Work out the finished part from the listing and answer in its coordinate system (mm). Face numbers are marked on the shaded views. A direction names the side the tool comes from. Round coordinates to 2 decimals unless told otherwise and drop trailing zeros. Loops run counter-clockwise (first coordinate to the right, second up) from the corner with the lowest first, then second, coordinate; pieces in that order, holes last. Notation, with made-up numbers: (-7.5, -6.75) - (21.5, -6.75) arc R26 cw to (21.5, 28.25) - close; hole circle Ø6 at (77, 3). An arc over 180 degrees is marked (long way). Answer as CSV lines item,"result". Start each with the question number.
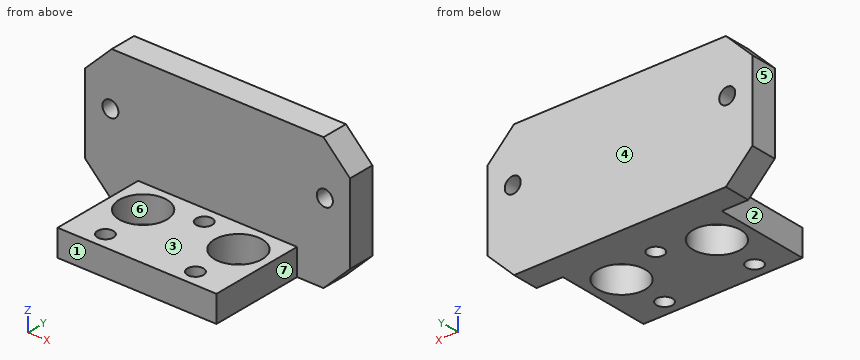
```python
from build123d import *

# Parameters (mm, degrees)
F0_R      = 1.51
F0_R_2    = 4.5
F1_DEPTH  = 5
F2_W      = 30
F2_H      = 5
F3_DEPTH  = 20
F4_W      = 5
F4_H      = 25
F5_DEPTH  = 10
F6_W      = 5
F6_H      = 25
F7_DEPTH  = 10
F9_DEPTH  = 5.001
F10_R     = 1.51
F11_DEPTH = 5.001


with BuildPart() as f1:
    # F0 (on Top) → F1 (new body)
    with BuildSketch(Plane.XY):
        Polygon((0, 18), (0, 0), (30, 0), (30, 18), (30, 23), (29.759806, 23), (0, 23), align=None)
        with Locations((6.5, 3)):
            Circle(F0_R, mode=Mode.SUBTRACT)
        with Locations((23.5, 3)):
            Circle(F0_R, mode=Mode.SUBTRACT)
        with Locations((6, 12)):
            Circle(F0_R_2, mode=Mode.SUBTRACT)
        with Locations((15, 15)):
            Circle(F0_R, mode=Mode.SUBTRACT)
        with Locations((24, 12)):
            Circle(F0_R_2, mode=Mode.SUBTRACT)
    extrude(amount=F1_DEPTH)

    # F2 (on face) → F3 (join)
    with BuildSketch(Plane.XY.offset(5)):
        with Locations((15, 20.5)):
            Rectangle(F2_W, F2_H)
    extrude(amount=F3_DEPTH)

    # F4 (on face) → F5 (join)
    with BuildSketch(Plane(origin=(0, 0, 0), x_dir=(0, -1, 0), z_dir=(-1, 0, 0))):
        with Locations((-20.5, 12.5)):
            Rectangle(F4_W, F4_H)
    extrude(amount=F5_DEPTH)

    # F6 (on face) → F7 (join)
    with BuildSketch(Plane.YZ.offset(30)):
        with Locations((20.5, 12.5)):
            Rectangle(F6_W, F6_H)
    extrude(amount=F7_DEPTH)

    # F8 (on face) → F9 (cut, through all)
    with BuildSketch(Plane.XZ.offset(-18)):
        Polygon((-5, 25), (-10, 25), (-10, 20), align=None)
        Polygon((-5, 0), (-10, 5), (-10, 0), align=None)
        Polygon((40, 5), (35, 0), (40, 0), align=None)
        Polygon((40, 25), (35, 25), (40, 20), align=None)
    extrude(amount=-F9_DEPTH, mode=Mode.SUBTRACT)

    # F10 (on face) → F11 (cut, through all)
    with BuildSketch(Plane.XZ.offset(-18)):
        with Locations((-5.25, 15)):
            Circle(F10_R)
        with Locations((35.25, 15)):
            Circle(F10_R)
    extrude(amount=-F11_DEPTH, mode=Mode.SUBTRACT)


solid = f1.part
```
Item 1: Section D-D, the plane y = 12 is taken. Give the vertices of the cut face in (x, z).
Item 2: Find the intervals of material crossed by L1, parallel to Z at x = 18.5, y = 11; L2, parallel to Y at x = -5, z = 10.75; L3, parallel to Z at x = -5.25, y = 21.3, in increasing order.
Item 3: Which of the six approach directions +Z, -Z, +X, -X, +Y, -Y give full straight-line access (tool end or side, diameter ignored) to the marked faces 1, 2 and 3?
Item 4: Determine the mould class of the marked faces 4, 5, 6 and 7 for opening direction X: pulls with the +X half, pulls with the -X half, needs draft (parallel to the pull), parting line crosses it, or undercut.
Item 5: Flat-ended cylindrical pins translate along their axes: pin 1 Ø1 at (x, y) = (1, 8) entering from +Z; pin 2 Ø4 at (y, z) = (8.5, 3.5) entering from +X; pin 3 Ø3.5 at (x, z) = (35.25, 15) entering from -Y. Find the tip coordinate at first contact, or state that the pin passes through.
Item 6: Section A-A, the plane z = 2.5 is taken. Give the vertices of the cut face in (x, y).
Item 7: Section C-C, the plane x = 24 is taken. Give the vertices of the cut face in (y, z).
Item 8: Section B-B, the plane y = 21.25 is taken. Give the vertices of the cut face in (x, z), and give its area (3 significant figures).
Answer:
1,outline,"(0, 0) - (1.5, 0) - (1.5, 5) - (0, 5) - close; (10.5, 0) - (19.5, 0) - (19.5, 5) - (10.5, 5) - close; (28.5, 0) - (30, 0) - (30, 5) - (28.5, 5) - close"
2,L1,"z = 0 to 5"
2,L2,"y = 18 to 23"
2,L3,"z = 0.25 to 13.49, 16.51 to 24.75"
3,face 1,"+Z, -Z, +X, -X, -Y"
3,face 2,"+Z, -Z, -X, -Y"
3,face 3,"+Z, +X, -X, -Y"
4,face 4,"needs draft"
4,face 5,"pulls with the -X half"
4,face 6,"undercut"
4,face 7,"pulls with the +X half"
5,pin 1,"stops at z = 5"
5,pin 2,"stops at x = 30"
5,pin 3,"stops at y = 18"
6,outline,"(-7.5, 18) - (0, 18) - (0, 0) - (30, 0) - (30, 18) - (37.5, 18) - (37.5, 23) - (-7.5, 23) - close; hole circle Ø9 at (6, 12); hole circle Ø3.02 at (6.5, 3); hole circle Ø3.02 at (15, 15); hole circle Ø9 at (24, 12); hole circle Ø3.02 at (23.5, 3)"
7,outline,"(0, 0) - (1.58, 0) - (1.58, 5) - (0, 5) - close; (4.42, 0) - (7.5, 0) - (7.5, 5) - (4.42, 5) - close; (16.5, 0) - (23, 0) - (23, 25) - (18, 25) - (18, 5) - (16.5, 5) - close"
8,outline,"(-10, 5) - (-5, 0) - (35, 0) - (40, 5) - (40, 20) - (35, 25) - (-5, 25) - (-10, 20) - close; hole circle Ø3.02 at (-5.25, 15); hole circle Ø3.02 at (35.25, 15)"
8,area,"1,190 mm²"
